For this review, take the finished solid that the model builds, in its own axes (mm). Face numbers are marked on the shaded views. Give positions to 0.01 mm unless a question says otherwise; leave off trailing zeros. Order: outer loops, then holes, each group sorted by start corner. A loop starts at its lowest first (then second) coordinate and runs counter-clockwise, first axis right, second up. Notation, with made-up numbers: (61, 74) - (116, 74) arc R18 ccw to (116, 93) - close; hole circle Ø4 at (76, 50). An arc over 180 degrees is marked (long way). Answer as a JSON object with one key per item and string values. Group by question number.
from build123d import *

# Parameters (mm, degrees)
BOSS_EXTRUDE1_DEPTH     = 38.1
SKETCH2_R               = 4.7625
SKETCH2_R_2             = 1.5875
BOSS_EXTRUDE3_DEPTH     = 2.409836439
CUT_EXTRUDE1_START      = -11.579198
CUT_EXTRUDE1_DEPTH      = 11.579198
SKETCH5_R               = 1.5875
CUT_EXTRUDE4_DEPTH      = 42.305774048
CUT_EXTRUDE5_REACH      = 43.306
CUT_EXTRUDE5_END_RADIUS = 44.104394081
SKETCH6_R               = 2


with BuildPart() as part:
    # Sketch1 → Boss-Extrude1 (new body)
    with BuildSketch(Plane(origin=(0, 0, 0), x_dir=(1, 0, 0), z_dir=(0, 1, 0))):
        with BuildLine():
            Line((-42.040163561, -13.335), (-35.690163561, -13.335))
            ThreePointArc((-35.690163561, -13.335), (-38.1, 0), (-35.690163561, 13.335))
            Line((-35.690163561, 13.335), (-42.040163561, 13.335))
            ThreePointArc((-42.040163561, 13.335), (-44.104394081, 0), (-42.040163561, -13.335))
        make_face()
    extrude(amount=BOSS_EXTRUDE1_DEPTH)

    # Sketch2 → Boss-Extrude3 (add)
    with BuildSketch(Plane.ZY.offset(42.040163561)):
        with Locations(Location((0, 30.070397704, 0), (0, 0, 180))):
            Circle(SKETCH2_R)
        with Locations(Location((0, 30.070397704, 0), (0, 0, 180))):
            Circle(SKETCH2_R_2, mode=Mode.SUBTRACT)
    extrude(amount=BOSS_EXTRUDE3_DEPTH)

    # Sketch3 → Cut-Extrude1 (cut)
    with BuildSketch(Plane.XZ.offset(CUT_EXTRUDE1_START)):
        with BuildLine():
            Line((-42.040163561, 13.335), (-35.690163561, 13.335))
            ThreePointArc((-35.690163561, 13.335), (-38.1, 0), (-35.690163561, -13.335))
            Line((-35.690163561, -13.335), (-42.040163561, -13.335))
            ThreePointArc((-42.040163561, -13.335), (-44.104394081, 0), (-42.040163561, 13.335))
        make_face()
    extrude(amount=CUT_EXTRUDE1_DEPTH, mode=Mode.SUBTRACT)

    # Sketch5 → Cut-Extrude4 (cut, through all)
    with BuildSketch(Plane.ZY.offset(44.45)):
        with Locations((0, 30.070397704)):
            Circle(SKETCH5_R)
    extrude(amount=-CUT_EXTRUDE4_DEPTH, mode=Mode.SUBTRACT)

    # Cut-Extrude5: up to this cylinder (the profile starts inside it)
    cut_extrude5_end = Plane(origin=(0, 22.450398, 0), z_dir=(0, -1, 0)) * Cylinder(CUT_EXTRUDE5_END_RADIUS, 175.820788161, mode=Mode.PRIVATE)
    # Sketch6 → Cut-Extrude5 (cut, up to the surface)
    with BuildSketch(Plane(origin=(-35.690163561, 0, 0), x_dir=(0, 0, -1), z_dir=(1, 0, 0)), mode=Mode.PRIVATE) as cut_extrude5_sk1:
        with Locations((0, 22.450397704)):
            Circle(SKETCH6_R)
    cut_extrude5_tool1 = extrude(cut_extrude5_sk1.sketch, amount=-CUT_EXTRUDE5_REACH, mode=Mode.PRIVATE) & cut_extrude5_end
    add(cut_extrude5_tool1.solids().sort_by_distance((-35.690164, 22.450398, 0))[0], mode=Mode.SUBTRACT)


solid = part.part
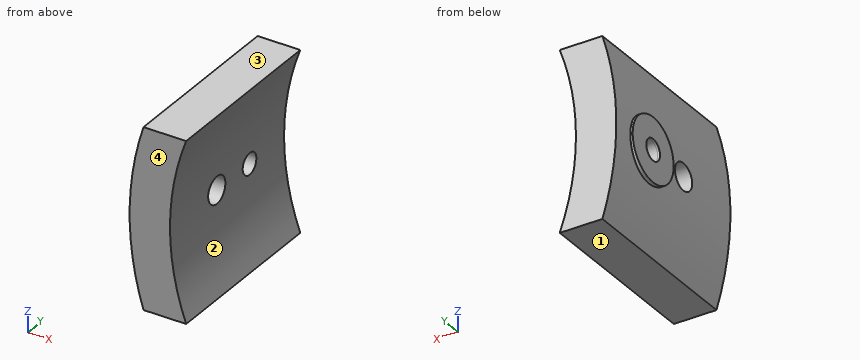
1) Consider section C-C (z = -3.5). Give the boundary of the cut face in (x, y).
2) For line 1 (Y direction, x = -39.5, z = 0); line 2 (Y direction, x = -44.25, z = 0); line 3 (Z direction, x = -39, y = 23.25) (3 decimals), list the stretches that pass through material, from the lowest coordinate up.
3) Consider section D-D (z = 7.75). Give the boundary of the cut face in (x, y), plus the area to 3 significant figures.
4) Mouldability with a two-part tool opening along Z and no side actions: class the marked faces 1, 2, 3 and 4 as released by +Z, released by -Z, zero draft, split by the parting line, or undercut.
5) Consider section A-A (z = 0). Give the boundary of the cut face in (x, y).
6) Consider section B-B (y = 18.25). Give the boundary of the cut face in (x, z) (3 decimals), plus the area to 3 significant figures.
7) For pin 1 (6.5 mm diameter, centred on y = 22.45, z = 0, fed in from +X); pin 2 (2.5 mm diameter, centred on y = 30.07, z = 0, fed in from -X); pin 3 (1 mm diameter, centred on y = 23.5, z = -7, fed in from +X); pin 4 (6 mm diameter, centred on y = 20.5, z = 7, fed in from -X), all flat-tipped, find the tip position at first contact; note any pin that passes through.
Result set:
{
 "1": {"outline": "(-44.45, 26.84) - (-43.97, 26.84) - (-43.97, 11.58) - (-37.94, 11.58) - (-37.94, 38.1) - (-43.97, 38.1) - (-43.97, 33.3) - (-44.45, 33.3) - close"},
 "2": {"line 1": "y = 11.58 to 20.45, 24.45 to 28.48, 31.66 to 38.1", "line 2": "y = 25.31 to 28.48, 31.66 to 34.83", "line 3": "z = -13.335 to -1.833, 1.833 to 13.335"},
 "3": {"outline": "(-43.42, 11.58) - (-37.3, 11.58) - (-37.3, 38.1) - (-43.42, 38.1) - close", "area": "162 mm2"},
 "4": {"face 1": "released by -Z", "face 2": "undercut", "face 3": "released by +Z", "face 4": "zero draft"},
 "5": {"outline": "(-44.45, 25.31) - (-44.1, 25.31) - (-44.1, 24.45) - (-38.1, 24.45) - (-38.1, 28.48) - (-44.45, 28.48) - close; (-44.45, 31.66) - (-38.1, 31.66) - (-38.1, 38.1) - (-44.1, 38.1) - (-44.1, 34.83) - (-44.45, 34.83) - close; (-44.1, 11.58) - (-38.1, 11.58) - (-38.1, 20.45) - (-44.1, 20.45) - close"},
 "6": {"outline": "(-42.04, -13.335) - (-35.69, -13.335) arc R38.1 cw to (-35.69, 13.335) - (-42.04, 13.335) arc R44.104 ccw to start", "area": "163 mm2"},
 "7": {"pin 1": "stops at x = -37.96", "pin 2": "passes through", "pin 3": "stops at x = -37.35", "pin 4": "stops at x = -43.92"}
}
